from build123d import *

# Parameters (mm, degrees)
RESSALTO_EXTRUS_O1_DEPTH   = 90
ESBO_O2_R                  = 5
CORTE_EXTRUS_O1_DEPTH      = 6
CORTE_EXTRUS_O2_DEPTH      = 101.031245119
CORTE_EXTRUS_O2_DEPTH_BACK = 101.031245119
ESBO_O3_R                  = 2
ESBO_O3_R_2                = 11.5
ESBO_O3_R_3                = 1.75
ESBO_O3_R_4                = 1.7
ESBO_O3_W                  = 25
ESBO_O3_H                  = 17
CORTE_EXTRUS_O4_START      = 8
ESBO_O4_W                  = 22.305447344
ESBO_O4_H                  = 5
ESBO_O4_W_2                = 48.791448981
CORTE_EXTRUS_O4_DEPTH      = 12
CORTE_EXTRUS_O7_REACH      = 103.253
ESBO_O6_R                  = 8
ESBO_O6_W                  = 20
ESBO_O6_H                  = 20
ESBO_O7_W                  = 4
ESBO_O7_H                  = 8
CORTE_EXTRUS_O8_DEPTH      = 102.253395156
ESBO_O11_R                 = 3.5
ESBO_O11_R_2               = 1.75
RESSALTO_EXTRUS_O3_DEPTH   = 12


with BuildPart() as part:
    # Esboço1 → Ressalto-extrusão1 (new body)
    with BuildSketch(Plane.XY):
        with BuildLine():
            Line((40, 0), (-40, 0))
            Line((-40, 0), (-40, -4))
            ThreePointArc((-40, -4), (-32.25, -11.75), (-40, -19.5))
            Line((-40, -19.5), (-40, -23.5))
            Line((-40, -23.5), (-30, -23.5))
            Line((-30, -23.5), (-22.205771366, -10))
            Line((-22.205771366, -10), (-4.683748499, -10))
            ThreePointArc((-4.683748499, -10), (0, -6.75), (4.683748499, -10))
            Line((4.683748499, -10), (22.205771366, -10))
            Line((22.205771366, -10), (30, -23.5))
            Line((30, -23.5), (40, -23.5))
            Line((40, -23.5), (40, -19.5))
            ThreePointArc((40, -19.5), (32.25, -11.75), (40, -4))
            Line((40, -4), (40, 0))
        make_face()
    extrude(amount=RESSALTO_EXTRUS_O1_DEPTH)

    # Esboço2 → Corte-extrusão1 (cut)
    with BuildSketch(Plane(origin=(0, 0, 0), x_dir=(1, 0, 0), z_dir=(0, 1, 0))):
        Polygon((-42.405591591, -59), (-12, -28.594408409), (18.405591591, -59), (-12, -89.405591591), align=None)
        with Locations(Location((-12, -59, 0), (0, 0, 270))):
            Circle(ESBO_O2_R, mode=Mode.SUBTRACT)
    extrude(amount=-CORTE_EXTRUS_O1_DEPTH, mode=Mode.SUBTRACT)

    # Esboço3 → Corte-extrusão2 (cut, two sides: drawn at the far end of the back side and taken through both)
    with BuildSketch(Plane(origin=(0, -6, 0), x_dir=(1, 0, 0), z_dir=(0, 1, 0)).offset(-CORTE_EXTRUS_O2_DEPTH_BACK)):
        with Locations(Location((-12, -37.079689783, 0), (0, 0, 180))):
            Circle(ESBO_O3_R)
        with Locations(Location((9.920310217, -59, 0), (0, 0, 180))):
            Circle(ESBO_O3_R)
        with Locations(Location((-12, -80.920310217, 0), (0, 0, 180))):
            Circle(ESBO_O3_R)
        with Locations(Location((-33.920310217, -59, 0), (0, 0, 180))):
            Circle(ESBO_O3_R)
        with Locations(Location((-12, -59, 0), (0, 0, 180))):
            Circle(ESBO_O3_R_2)
        with Locations(Location((-30, -42, 0), (0, 0, 180))):
            Circle(ESBO_O3_R_3)
        with Locations(Location((10, -42, 0), (0, 0, 180))):
            Circle(ESBO_O3_R_3)
        with Locations(Location((-17.5, -12, 0), (0, 0, 180))):
            Circle(ESBO_O3_R_4)
        with Locations(Location((17.5, -12, 0), (0, 0, 180))):
            Circle(ESBO_O3_R_4)
        with Locations(Location((17, -75, 0), (0, 0, 180))):
            Circle(ESBO_O3_R_3)
        with Locations(Location((-13, -25, 0), (0, 0, 180))):
            Circle(ESBO_O3_R_3)
        with Locations(Location((17, -25, 0), (0, 0, 180))):
            Circle(ESBO_O3_R_3)
        with Locations((0, -8.5)):
            Rectangle(ESBO_O3_W, ESBO_O3_H)
    extrude(amount=CORTE_EXTRUS_O2_DEPTH + CORTE_EXTRUS_O2_DEPTH_BACK, mode=Mode.SUBTRACT)

    # Esboço4 → Corte-extrusão4 (cut)
    with BuildSketch(Plane.XZ.offset(10).offset(CORTE_EXTRUS_O4_START)):
        with BuildLine():
            Line((-13.998411754, 37), (-22.205771366, 37))
            Line((-22.205771366, 37), (-22.205771366, 32))
            Line((-22.205771366, 32), (-4.683748499, 32))
            Line((-4.683748499, 32), (-4.683748499, 37))
            Line((-4.683748499, 37), (-10.001588246, 37))
            ThreePointArc((-10.001588246, 37), (-12, 35.079689783), (-13.998411754, 37))
        make_face()
        with Locations((-33.358495038, 34.5)):
            Rectangle(ESBO_O4_W, ESBO_O4_H)
        with Locations((19.711975992, 34.5)):
            Rectangle(ESBO_O4_W_2, ESBO_O4_H)
    extrude(amount=CORTE_EXTRUS_O4_DEPTH, mode=Mode.SUBTRACT)

    # Corte-extrusão7: up to this face of the body (flat: up to its plane)
    corte_extrus_o7_end = Plane(part.part.faces().sort_by_distance((-13.702636596, -10, 79.456396835))[0])
    # Esboço6 → Corte-extrusão7 (cut, up to the picked face)
    with BuildSketch(Plane.XZ.offset(23.5), mode=Mode.PRIVATE) as corte_extrus_o7_sk1:
        with Locations((17, 75)):
            Circle(ESBO_O6_R)
    corte_extrus_o7_tool1 = split(extrude(corte_extrus_o7_sk1.sketch, amount=-CORTE_EXTRUS_O7_REACH, mode=Mode.PRIVATE), bisect_by=corte_extrus_o7_end, keep=Keep.BOTH, mode=Mode.PRIVATE)
    # Esboço6 → Corte-extrusão7 (cut, up to the picked face)
    with BuildSketch(Plane.XZ.offset(23.5), mode=Mode.PRIVATE) as corte_extrus_o7_sk2:
        with Locations((17, 25)):
            Circle(ESBO_O6_R)
    corte_extrus_o7_tool2 = split(extrude(corte_extrus_o7_sk2.sketch, amount=-CORTE_EXTRUS_O7_REACH, mode=Mode.PRIVATE), bisect_by=corte_extrus_o7_end, keep=Keep.BOTH, mode=Mode.PRIVATE)
    # Esboço6 → Corte-extrusão7 (cut, up to the picked face)
    with BuildSketch(Plane.XZ.offset(23.5), mode=Mode.PRIVATE) as corte_extrus_o7_sk3:
        with Locations((-13, 25)):
            Circle(ESBO_O6_R)
    corte_extrus_o7_tool3 = split(extrude(corte_extrus_o7_sk3.sketch, amount=-CORTE_EXTRUS_O7_REACH, mode=Mode.PRIVATE), bisect_by=corte_extrus_o7_end, keep=Keep.BOTH, mode=Mode.PRIVATE)
    # Esboço6 → Corte-extrusão7 (cut, up to the picked face)
    with BuildSketch(Plane.XZ.offset(23.5), mode=Mode.PRIVATE) as corte_extrus_o7_sk4:
        with Locations((-30, 42)):
            Rectangle(ESBO_O6_W, ESBO_O6_H)
    corte_extrus_o7_tool4 = split(extrude(corte_extrus_o7_sk4.sketch, amount=-CORTE_EXTRUS_O7_REACH, mode=Mode.PRIVATE), bisect_by=corte_extrus_o7_end, keep=Keep.BOTH, mode=Mode.PRIVATE)
    add(corte_extrus_o7_tool1.solids().sort_by(Axis((17, -23.5, 75), (0, 1, 0)))[0], mode=Mode.SUBTRACT)
    add(corte_extrus_o7_tool2.solids().sort_by(Axis((17, -23.5, 25), (0, 1, 0)))[0], mode=Mode.SUBTRACT)
    add(corte_extrus_o7_tool3.solids().sort_by(Axis((-13, -23.5, 25), (0, 1, 0)))[0], mode=Mode.SUBTRACT)
    add(corte_extrus_o7_tool4.solids().sort_by(Axis((-30, -23.5, 42), (0, 1, 0)))[0], mode=Mode.SUBTRACT)

    # Esboço7 → Corte-extrusão8 (cut, through all)
    with BuildSketch(Plane(origin=(0, 0, 0), x_dir=(1, 0, 0), z_dir=(0, 1, 0))):
        with Locations((27.000875928, -80)):
            Rectangle(ESBO_O7_W, ESBO_O7_H)
        with Locations((27.000875928, -10)):
            Rectangle(ESBO_O7_W, ESBO_O7_H)
        with Locations((-27.000875928, -10)):
            Rectangle(ESBO_O7_W, ESBO_O7_H)
        with Locations((-27.000875928, -80)):
            Rectangle(ESBO_O7_W, ESBO_O7_H)
    extrude(amount=-CORTE_EXTRUS_O8_DEPTH, mode=Mode.SUBTRACT)

    # Esboço11 → Ressalto-extrusão3 (add)
    # profile 1 of 3: a face of its own
    with BuildSketch(Plane.XZ.offset(10)):
        with Locations(Location((-13, 25, 0), (0, 0, 180))):
            Circle(ESBO_O11_R)
        with Locations(Location((-13, 25, 0), (0, 0, 180))):
            Circle(ESBO_O11_R_2, mode=Mode.SUBTRACT)
    # profile 2 of 3: a face of its own
    with BuildSketch(Plane.XZ.offset(10)):
        with Locations(Location((17, 25, 0), (0, 0, 180))):
            Circle(ESBO_O11_R)
        with Locations(Location((17, 25, 0), (0, 0, 180))):
            Circle(ESBO_O11_R_2, mode=Mode.SUBTRACT)
    # profile 3 of 3: a face of its own
    with BuildSketch(Plane.XZ.offset(10)):
        with Locations(Location((17, 75, 0), (0, 0, 180))):
            Circle(ESBO_O11_R)
        with Locations(Location((17, 75, 0), (0, 0, 180))):
            Circle(ESBO_O11_R_2, mode=Mode.SUBTRACT)
    extrude(amount=RESSALTO_EXTRUS_O3_DEPTH)


solid = part.part
Check sheet for the modelled part. Datum: model origin and axes. Units: mm. A direction names the side the tool comes from. Give positions to 0.01 mm unless a question says otherwise; leave off trailing zeros. Write each loop counter-clockwise with the first axis right and the second up, starting at its lowest first coordinate (ties: lowest second). Pieces come first, ordered by that corner, then holes. Notation, with made-up numbers: (-24, -10.5) -> (-14, -10.5) arc R31 ccw to (-14, 26.5) -> close; hole circle Ø11 at (19, 57). An arc over 180 degrees is marked (long way). One line per item, written item: value. Start each with the question number.
Item 1: Draft check along Z on faces 5 (the cylindrical face through (-12.54, -15.92, 21.53)), 6 (the flat face through (9, 0, 44)), 7 (the flat face through (27, -8, 14)). Enter one of: +Z half, -Z half, draft (parallel to the pull), parting line (faces both ways), or undercut.
Item 2: Gauge pin test, flat ends, axial feed: pin 1 (5.5 mm diameter, centred on x = 10, z = 42, fed in from -Y); pin 2 (6.5 mm diameter, centred on x = 9.92, z = 59, fed in from +Y); pin 3 (7.5 mm diameter, centred on x = 18, z = 76.5, fed in from -Y); pin 4 (3 mm diameter, centred on x = 17.5, z = 12, fed in from -Y). Record the tip position at first contact, or that the pin passes through.
Item 3: Tool access check on faces 1 (the cylindrical face through (25, -12, 75)), 2 (the flat face through (19, -22, 76)), 3 (the flat face through (-26.196, -2.958, 42.79)), 4 (the flat face through (27, -8, 76)). Record the directions out of +Z, -Z, +X, -X, +Y, -Y that give a thin tool (end or side, any length) a straight path to the whole face; none if there is none.
Item 4: Section check A-A on z = 25. State how many separate pieces and enclosed holes the cut face has, then the cut area to 3 significant figures.
Item 5: Material ranges on probe 1 along Z at (x, y) = (27.5, -13.5); probe 2 along X at (y, z) = (-20.25, 13); probe 3 along Z at (x, y) = (-13, -15.5), recorded low to high. Write a range as from..to.
Item 6: Section check C-C on x = -17.5. Record the cut outline in (y, z), then the cut area to 3 significant figures.
Item 7: Section check B-B on x = 17. Record the cut outline in (y, z).
Results list:
1. face 5: parting line
1. face 6: draft
1. face 7: undercut
2. pin 1: y = -10
2. pin 2: y = -6
2. pin 3: y = -22
2. pin 4: through
3. face 1: -Y
3. face 2: +Z, -Z, -Y
3. face 3: +Y
3. face 4: +Y, -Y
4. separate pieces: 3
4. enclosed holes: 0
4. area: 972 mm²
5. probe 1: 0..6, 14..76, 84..90
5. probe 2: -40..-29, 29..40
5. probe 3: 21.5..23.25, 26.75..28.5
6. outline: (-10, 0) -> (0, 0) -> (0, 10.3) -> (-10, 10.3) -> close; (-10, 13.7) -> (0, 13.7) -> (0, 34.09) -> (-6, 34.09) -> (-6, 48.9) -> (-10, 48.9) -> close; (-10, 69.1) -> (-6, 69.1) -> (-6, 83.91) -> (0, 83.91) -> (0, 90) -> (-10, 90) -> close
6. area: 486 mm²
7. outline: (-22, 21.5) -> (-10, 21.5) -> (-10, 13.62) -> (0, 13.62) -> (0, 23.25) -> (-22, 23.25) -> close; (-22, 26.75) -> (0, 26.75) -> (0, 57.59) -> (-6, 57.59) -> (-6, 60.41) -> (0, 60.41) -> (0, 73.25) -> (-22, 73.25) -> (-22, 71.5) -> (-10, 71.5) -> (-10, 28.5) -> (-22, 28.5) -> close; (-22, 76.75) -> (0, 76.75) -> (0, 90) -> (-10, 90) -> (-10, 78.5) -> (-22, 78.5) -> close; (-10, 0) -> (0, 0) -> (0, 10.38) -> (-10, 10.38) -> close
